Verification items for this drawing (mm, ordinates from the low corner). Coordinates: 2 decimals unless noted, no trailing zeros. Order: outer loops, then holes, each group sorted by start corner. A loop starts at its lowest first (then second) coordinate and runs counter-clockwise, first axis right, second up.
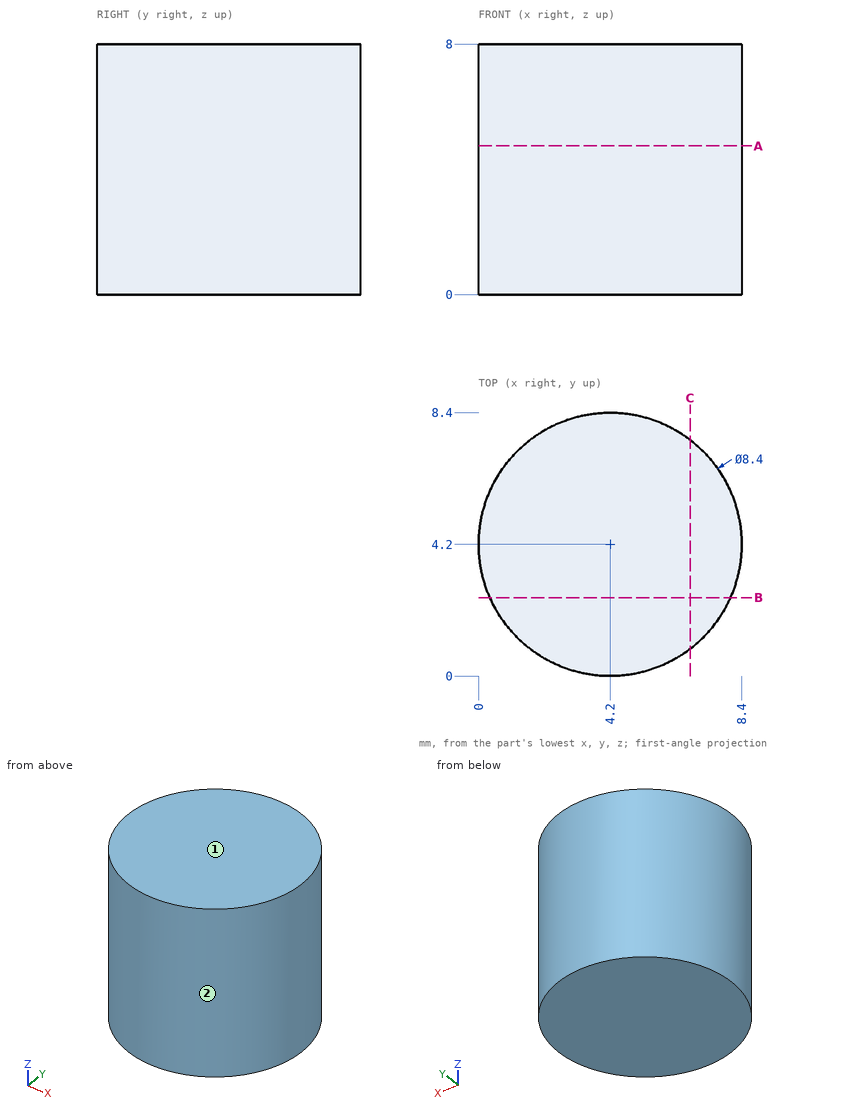
(1) Thickness scan on probe 1 along X at (y, z) = (3, 4.75); probe 2 along X at (y, z) = (6, 5.25); probe 3 along Y at (x, z) = (5.5, 7.25). Record the ranges inside material, lowest first.
Filled in:
probe 1: x = 0.18 to 8.22
probe 2: x = 0.41 to 7.99
probe 3: y = 0.21 to 8.19
(2) Go/stop test with flat-tipped pins: P1, Ø3, axis at x = 6, z = 7, coming from the -Y side; P2, Ø1, axis at y = 7, z = 5, coming from the +X side; P3, Ø1, axis at x = 1.5, z = 6.5, coming from the -Y side. Record where each tip stops, or that it passes through.
Filled in:
P1: stops at y = 0.01
P2: stops at x = 7.71
P3: stops at y = 0.62
(3) Cross-section at C-C (x = 6.75). Enter the section's corners in (y, z).
Filled in:
outline: (0.86, 0) - (7.54, 0) - (7.54, 8) - (0.86, 8) - close
(4) Cross-section at A-A (z = 4.75). Enter the section's corners in (x, y), and give its area (3 significant figures).
Filled in:
outline: circle Ø8.4 at (4.2, 4.2)
area: 55.4 mm2
(5) Cross-section at B-B (y = 2.5). Enter the section's corners in (x, z).
Filled in:
outline: (0.36, 0) - (8.04, 0) - (8.04, 8) - (0.36, 8) - close
(6) Release check for a two-part mould opening along X. For the marked faces 1 and 2 record: +X half, -X half, draft (parallel to the pull), parting line (faces both ways), or undercut.
Filled in:
face 1: draft
face 2: parting line
